The listing builds one solid part. Answer for the finished solid, in the listing's coordinates (mm). Face numbers are marked on the shaded views. Give positions to 0.01 mm unless a question says otherwise; leave off trailing zeros. Order: outer loops, then holes, each group sorted by start corner. A loop starts at its lowest first (then second) coordinate and runs counter-clockwise, first axis right, second up. Notation, with made-up numbers: (26.5, 61) - (70.5, 61) arc R31 ccw to (70.5, 86) - close; hole circle Ø5 at (9.25, 79). An arc over 180 degrees is marked (long way). Answer in a Markdown table with one row per item.
Autodesk Inventor part; units mm, degrees
ref_plane "YZ Plane" through (0, 0, 0) normal (1, 0, 0) x (0, 1, 0)
ref_plane "XZ Plane" through (0, 0, 0) normal (0, 1, 0) x (-1, 0, 0)
ref_plane "XY Plane" through (0, 0, 0) normal (0, 0, 1) x (1, 0, 0)
sketch "Sketch1" plane through (0, 0, 0) normal (0, 0, 1) x (1, 0, 0)
  circle A0 centre (0, 0) radius 32
  dimension "d0" = 64
extrude "Extrusion1" add sketch "Sketch1" along normal blind 2
sketch "Sketch2" plane through (0, 0, 2) normal (0, 0, 1) x (1, 0, 0)
  line L0 (0, 0) -> (0, 32) construction
  circle A0 centre (0, 0) radius 32 construction
  arc A1 (-0.9, 30.658) -> (0.9, 30.658) centre (0, 30.658) ccw
  line L1 (-0.9, 30.658) -> (-0.9, 31.9873)
  line L2 (0.9, 30.658) -> (0.9, 31.9873)
  circle A2 centre (0, 0) radius 32
  arc A3 (0.9, 31.9873) -> (-0.9, 31.9873) centre (0, 0) ccw
  arc A4 (-26.1006, -16.1084) -> (-27.0006, -14.5496) centre (-26.5506, -15.329) ccw
  line L3 (-26.1006, -16.1084) -> (-27.2519, -16.7731)
  line L4 (-27.0006, -14.5496) -> (-28.1519, -15.2142)
  arc A5 (-28.1519, -15.2142) -> (-27.2519, -16.7731) centre (0, 0) ccw
  arc A6 (27.0006, -14.5496) -> (26.1006, -16.1084) centre (26.5506, -15.329) ccw
  line L5 (27.0006, -14.5496) -> (28.1519, -15.2142)
  line L6 (26.1006, -16.1084) -> (27.2519, -16.7731)
  arc A7 (27.2519, -16.7731) -> (28.1519, -15.2142) centre (0, 0) ccw
  point P0 (-27.7128, -16)
  point P1 (27.7128, -16)
  dimension "d3" = 30.658
  dimension "d4" = 1.8
  dimension "d7" = 360
extrude "Extrusion2" cut sketch "Sketch2" against normal through all contours L1 A2 L2 A1 | L4 A4 L3 A2 | A2 L6 A6 L5
sketch "Sketch3" plane through (0, 0, 2) normal (0, 0, 1) x (1, 0, 0)
  line L0 (22.9, -4.5) -> (25.1, -4.5)
  line L1 (25.1, -4.5) -> (25.1, 4.5)
  line L2 (25.1, 4.5) -> (22.9, 4.5)
  line L3 (22.9, 4.5) -> (22.9, -4.5)
  line L4 (22.9, -4.5) -> (25.1, 4.5) construction
  line L5 (25.1, -4.5) -> (22.9, 4.5) construction
  circle A0 centre (0, 0) radius 28.815 construction
  point P0 (24, 0)
  dimension "d11" = 2.2
  dimension "d12" = 9
  dimension "d21" = 57.63
  dimension "d22" = 24
extrude "Extrusion3" cut sketch "Sketch3" against normal through all
sketch "Sketch4" plane through (0, 0, 2) normal (0, 0, 1) x (1, 0, 0)
  line L0 (25.1, 4.5) -> (25.1, -4.5)
  line L1 (25.1, -4.5) -> (22.9, -4.5)
  line L2 (22.9, -4.5) -> (22.9, 4.5)
  line L3 (22.9, 4.5) -> (25.1, 4.5)
  line L4 (-26.1006, -16.1084) -> (-27.2519, -16.7731)
  arc A0 (-27.2519, -16.7731) -> (27.2519, -16.7731) centre (0, 0) ccw
  line L5 (27.2519, -16.7731) -> (26.1006, -16.1084)
  arc A1 (27.0006, -14.5496) -> (26.1006, -16.1084) centre (26.5506, -15.329) ccw
  line L6 (27.0006, -14.5496) -> (28.1519, -15.2142)
  arc A2 (28.1519, -15.2142) -> (0.9, 31.9873) centre (0, 0) ccw
  line L7 (0.9, 31.9873) -> (0.9, 30.658)
  arc A3 (-0.9, 30.658) -> (0.9, 30.658) centre (0, 30.658) ccw
  line L8 (-0.9, 30.658) -> (-0.9, 31.9873)
  arc A4 (-0.9, 31.9873) -> (-28.1519, -15.2142) centre (0, 0) ccw
  line L9 (-28.1519, -15.2142) -> (-27.0006, -14.5496)
  arc A5 (-26.1006, -16.1084) -> (-27.0006, -14.5496) centre (-26.5506, -15.329) ccw
  line L10 (22.9, -4.5) -> (22.9, 4.5)
  line L11 (22.9, 0) -> (25.1, 0) construction
  arc A6 (22.9, 3.5) -> (22.9, 2.5) centre (22.9, 3) ccw
  arc A7 (22.9, -2.5) -> (22.9, -3.5) centre (22.9, -3) ccw
  line L12 (22.9, -2.5) -> (22.9, -3.5)
  line L13 (22.9, 3.5) -> (22.9, 2.5)
  dimension "d15" = 3
  dimension "d16" = 3
  dimension "d17" = 1
  dimension "d18" = 1
extrude "Extrusion4" cut sketch "Sketch4" against normal blind 1 contours L2 A6 | A7 L2
sketch "Sketch5" plane through (0, 0, 0) normal (0, 0, -1) x (-1, 0, 0)
  line L0 (-25.1, -4.5) -> (-25.1, 4.5)
  line L1 (-25.1, 4.5) -> (-22.9, 4.5)
  line L2 (-22.9, 4.5) -> (-22.9, -4.5)
  line L3 (-22.9, -4.5) -> (-25.1, -4.5)
  line L4 (27.2519, -16.7731) -> (26.1006, -16.1084)
  arc A0 (27.0006, -14.5496) -> (26.1006, -16.1084) centre (26.5506, -15.329) ccw
  line L5 (27.0006, -14.5496) -> (28.1519, -15.2142)
  arc A1 (28.1519, -15.2142) -> (0.9, 31.9873) centre (0, 0) ccw
  line L6 (0.9, 31.9873) -> (0.9, 30.658)
  arc A2 (-0.9, 30.658) -> (0.9, 30.658) centre (0, 30.658) ccw
  line L7 (-0.9, 30.658) -> (-0.9, 31.9873)
  arc A3 (-0.9, 31.9873) -> (-28.1519, -15.2142) centre (0, 0) ccw
  line L8 (-28.1519, -15.2142) -> (-27.0006, -14.5496)
  arc A4 (-26.1006, -16.1084) -> (-27.0006, -14.5496) centre (-26.5506, -15.329) ccw
  line L9 (-26.1006, -16.1084) -> (-27.2519, -16.7731)
  arc A5 (-27.2519, -16.7731) -> (27.2519, -16.7731) centre (0, 0) ccw
  line L10 (-22.9, 4.5) -> (-25.1, 4.5)
  line L11 (-25.1, 4.5) -> (-25.1, -4.5)
  line L12 (-25.1, -4.5) -> (-22.9, -4.5)
  line L13 (-22.9, -4.5) -> (-22.9, 4.5)
  line L14 (-22.9, 4.5) -> (-25.1, -4.5) construction
  line L15 (-25.1, 4.5) -> (-22.9, -4.5) construction
  line L16 (-20.9, 6.5) -> (-27.1, 6.5)
  line L17 (-27.1, 6.5) -> (-27.1, -6.5)
  line L18 (-27.1, -6.5) -> (-20.9, -6.5)
  line L19 (-20.9, -6.5) -> (-20.9, 6.5)
  circle A6 centre (0, 0) radius 28.815 construction
  point P0 (-24, 0)
  dimension "d23" = 2
  dimension "d24" = 57.63
extrude "Extrusion5" add sketch "Sketch5" along normal blind 2 contours L19 L18 L17 L16
sketch "Sketch6" plane through (0, 0, 0) normal (0, 1, 0) x (-1, 0, 0)
  line L0 (0, 0) -> (-15.5, 0) construction
  line L1 (-27.2519, 0) -> (27.2519, 0)
  line L2 (-15.5, 0) -> (-17.5, 0)
  line L3 (-17.5, 0) -> (-17.5, -8.5)
  line L4 (-17.5, -8.5) -> (-9, -8.5)
  line L5 (-9, -8.5) -> (-9, -6.5)
  line L6 (-9, -6.5) -> (-15.5, -6.5)
  line L7 (-15.5, -6.5) -> (-15.5, 0)
  line L8 (0, 0) -> (0, -14.0631) construction
  line L9 (15.5, 0) -> (17.5, 0)
  line L10 (17.5, 0) -> (17.5, -8.5)
  line L11 (17.5, -8.5) -> (9, -8.5)
  line L12 (9, -8.5) -> (9, -6.5)
  line L13 (9, -6.5) -> (15.5, -6.5)
  line L14 (15.5, -6.5) -> (15.5, 0)
  dimension "d27" = 15.5
  dimension "d28" = 2
  dimension "d29" = 8.5
  dimension "d30" = 8.5
  dimension "d31" = 2
extrude "Extrusion6" add sketch "Sketch6" along normal mid plane 16
fillet "Fillet1" radius 2 1 edges at (-17.5, 0, -8.5)
fillet "Fillet2" radius 2 1 edges at (17.5, 0, -8.5)
properties part number "joint_lid" material "Acetal Resin, Black"
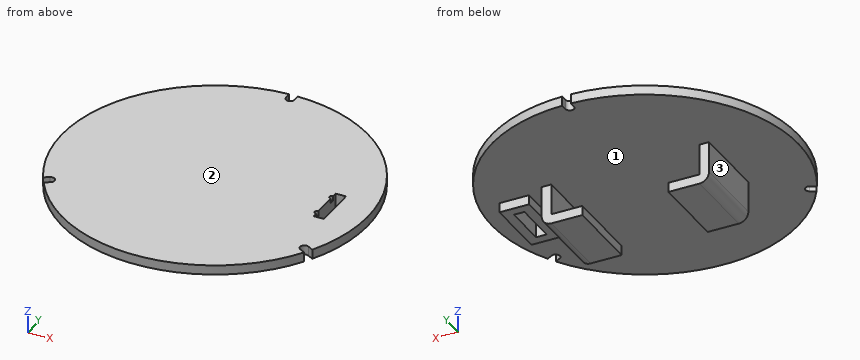
Item 1: Each of these flat-tipped pins is pushed along its axis until it touches: P1, Ø3, axis at x = -17.5, z = -2.5, coming from the -Y side; P2, Ø1.6, axis at y = 1, z = -1, coming from the +X side; P3, Ø2, axis at y = -1, z = -1.5, coming from the -X side; P4, Ø10, axis at x = -7.5, y = 6.5, coming from the -Z side. Where does it stop, or does it pass through?
Answer block:
| item | result |
|---|---|
| P1 | y = -8 |
| P2 | x = 27.1 |
| P3 | x = -17.5 |
| P4 | z = -8.5 |
Item 2: Determine the mould class of the marked faces 1, 2 and 3 for opening direction X: pulls with the +X half, pulls with the -X half, needs draft (parallel to the pull), parting line crosses it, or undercut.
Answer block:
| item | result |
|---|---|
| face 1 | undercut |
| face 2 | needs draft |
| face 3 | pulls with the -X half |
Item 3: Find section C-C on x = 0. Write down the section's boundary in (y, z), then the cut area to 3 significant figures.
Answer block:
| item | result |
|---|---|
| outline | (-32, 0) - (29.76, 0) - (29.76, 2) - (-32, 2) - close |
| area | 124 mm² |
Item 4: Consider line 1 (X direction, y = -1.5, z = -0.5); line 2 (X direction, y = 0.5, z = -6.25); line 3 (Z direction, x = 7, y = 3). Determine where each line is inside the solid, lowest interval first.
Answer block:
| item | result |
|---|---|
| line 1 | -17.5 to -15.5, 15.5 to 17.5, 20.9 to 22.9, 25.1 to 27.1 |
| line 2 | -17.5 to -15.5, 15.5 to 17.5 |
| line 3 | 0 to 2 |
Item 5: Find section B-B on z = -3.5. Write down the section's boundary in (x, y).
Answer block:
| item | result |
|---|---|
| outline | (-17.5, -8) - (-15.5, -8) - (-15.5, 8) - (-17.5, 8) - close; (15.5, -8) - (17.5, -8) - (17.5, 8) - (15.5, 8) - close |
Item 6: Find section D-D on y = -10.5. Write down the section's boundary in (x, z).
Answer block:
| item | result |
|---|---|
| outline | (-30.23, 0) - (30.23, 0) - (30.23, 2) - (-30.23, 2) - close |
Item 7: Find section A-A on y = 0. Write down the section's boundary in (x, z), then the cut area to 3 significant figures.
Answer block:
| item | result |
|---|---|
| outline | (-32, 0) - (-17.5, 0) - (-17.5, -6.5) arc R2 ccw to (-15.5, -8.5) - (-9, -8.5) - (-9, -6.5) - (-15.5, -6.5) - (-15.5, 0) - (15.5, 0) - (15.5, -6.5) - (9, -6.5) - (9, -8.5) - (15.5, -8.5) arc R2 ccw to (17.5, -6.5) - (17.5, 0) - (20.9, 0) - (20.9, -2) - (22.9, -2) - (22.9, 2) - (-32, 2) - close; (25.1, -2) - (27.1, -2) - (27.1, 0) - (32, 0) - (32, 2) - (25.1, 2) - close |
| area | 190 mm² |
